Source: three-view drawing plus pictorial views. Frame: mm from the lowest corner of the part. A direction names the side the tool comes from. Give positions to 0.01 mm unless a question says otherwise; leave off trailing zeros. Write each loop counter-clockwise with the first axis right and the second up, starting at its lowest first coordinate (ties: lowest second). Pieces come first, ordered by that corner, then holes.
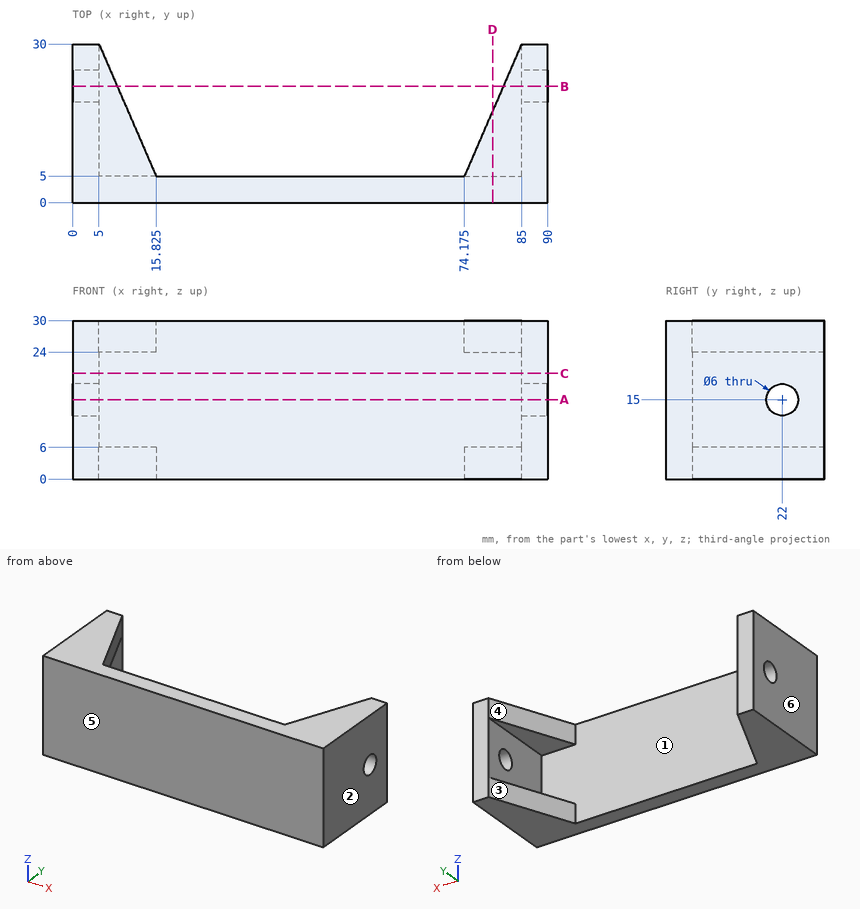
Q1. Section C-C on z = 20. Output: boundary loops of the cut face in (x, y), plus the area to 3 significant figures.
Filled sheet:
outline: (0, 0) - (90, 0) - (90, 30) - (85, 30) - (85, 5) - (5, 5) - (5, 30) - (0, 30) - close
area: 700 mm2
Q2. Access query for the marked faces 1, 2 and 3. Directions: +Z, -Z, +X, -X, +Y, -Y. A direction counts if a zero-diameter tool reaches every point of the face in a straight line with its end or side. Return the directions, or none.
Filled sheet:
face 1: +Y
face 2: +Z, -Z, +X, +Y, -Y
face 3: +Z, -Z, +Y
Q3. Pin query (flat end, axial travel): P1, Ø10, axis at x = 63.5, z = 24.5, coming from the -Y side; P2, Ø15, axis at x = 26, z = 12, coming from the +Y side; P3, Ø5, axis at y = 22, z = 15, coming from the -X side (1 decimal). Return the tip coordinate at first contact, or that it passes through.
Filled sheet:
P1: stops at y = 0
P2: stops at y = 5
P3: passes through
Q4. Section B-B on y = 22. Output: boundary loops of the cut face in (x, z), plus the area to 3 significant figures.
Filled sheet:
outline: (0, 0) - (8.46, 0) - (8.46, 6) - (5, 6) - (5, 12) - (0, 12) - close; (0, 18) - (5, 18) - (5, 24) - (8.46, 24) - (8.46, 30) - (0, 30) - close; (81.54, 0) - (90, 0) - (90, 12) - (85, 12) - (85, 6) - (81.54, 6) - close; (81.54, 24) - (85, 24) - (85, 18) - (90, 18) - (90, 30) - (81.54, 30) - close
area: 323 mm2
Q5. Section D-D on x = 79.5. Output: boundary loops of the cut face in (y, z), plus the area to 3 significant figures.
Filled sheet:
outline: (0, 0) - (17.3, 0) - (17.3, 6) - (5, 6) - (5, 24) - (17.3, 24) - (17.3, 30) - (0, 30) - close
area: 298 mm2
Q6. Section A-A on z = 15. Output: boundary loops of the cut face in (x, y).
Filled sheet:
outline: (0, 0) - (90, 0) - (90, 19) - (85, 19) - (85, 5) - (5, 5) - (5, 19) - (0, 19) - close; (0, 25) - (5, 25) - (5, 30) - (0, 30) - close; (85, 25) - (90, 25) - (90, 30) - (85, 30) - close
Q7. Ray query, line 1 along Z through (x, y) = (3, 22); line 2 along X through (y, z) = (13, 15.25); line 3 along Y through (x, z) = (86.85, 15). Return the intervals inside material, ascending.
Filled sheet:
line 1: z = 0 to 12, 18 to 30
line 2: x = 0 to 5, 85 to 90
line 3: y = 0 to 19, 25 to 30
Q8. Pull-direction query (X, two-part tool) for the marked faces 4, 5 and 6; classes: released by +X, released by -X, zero draft, split by the parting line, or undercut.
Filled sheet:
face 4: undercut
face 5: zero draft
face 6: released by -X
